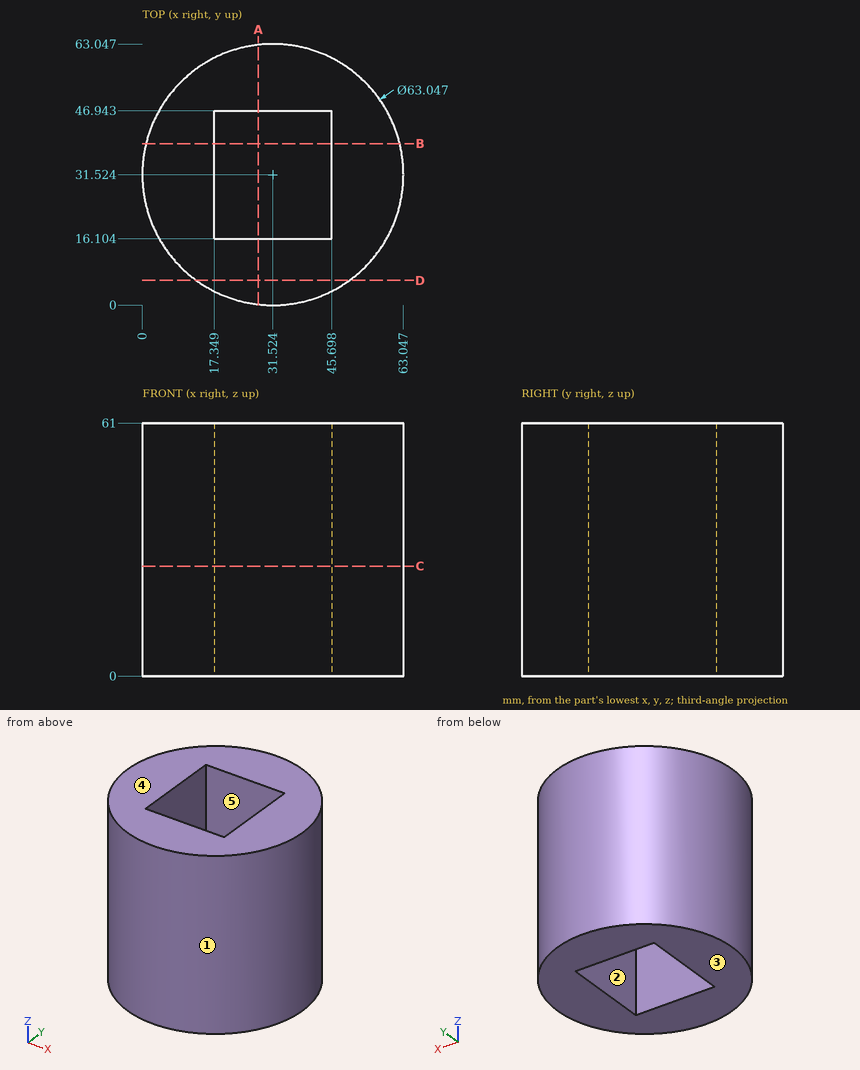
The figure shows three views and two pictorial views of one solid part (mm, origin at its lowest corner). Answer the questions. A direction names the side the tool comes from. Give positions to 0.01 mm unless a question says otherwise; leave off trailing zeros. Write each loop counter-clockwise with the first axis right and the second up, starting at its lowest first coordinate (ties: lowest second). Pieces come first, ordered by that corner, then holes.
Q1. For a pull along Y with two mould halves and no side action, classify the marked faces 1, 2 and 3 as released by +Y, released by -Y, zero draft, split by the parting line, or undercut.
Answer:
face 1: split by the parting line
face 2: undercut
face 3: zero draft
Q2. The part is cut by section B-B on y = 39. Give the vertices of the cut face in (x, z).
Answer:
outline: (0.9, 0) - (17.35, 0) - (17.35, 61) - (0.9, 61) - close; (45.7, 0) - (62.15, 0) - (62.15, 61) - (45.7, 61) - close
Q3. Given pin 1 (6 mm diameter, centred on x = 28, z = 30.5, fed in from -Y); pin 2 (2 mm diameter, centred on x = 53, y = 6.5, fed in from +Z); pin 3 (8.5 mm diameter, centred on x = 28.5, z = 24, fed in from +Y); pin 4 (1 mm diameter, centred on y = 56.5, z = 32, fed in from -X), each flat-ended and moving along its own axis, determine where each tip first touches the part or whether it passes through.
Answer:
pin 1: stops at y = 0
pin 2: passes through
pin 3: stops at y = 63.05
pin 4: stops at x = 11.66
Q4. Straight lines are drawn through the part: L1, parallel to Y at x = 39.5, z = 17.5 (1 decimal); L2, parallel to X at y = 8, z = 46.5; L3, parallel to X at y = 28, z = 3. For each, find the intervals that lie inside material, in ascending order.
Answer:
L1: y = 1 to 16.1, 46.9 to 62
L2: x = 10.54 to 52.51
L3: x = 0.2 to 17.35, 45.7 to 62.85
Q5. The part is cut by section C-C on z = 26.5. Give the vertices of the cut face in (x, y).
Answer:
outline: circle Ø63.05 at (31.52, 31.52); hole (17.35, 16.1) - (45.7, 16.1) - (45.7, 46.94) - (17.35, 46.94) - close
Q6. A tool of negligible diameter and unlimited length cuts with its end or side. For the marked faces 4 and 5, from which of +Z, -Z, +X, -X, +Y, -Y can it reach the whole face along a straight path? Write none if from no direction.
Answer:
face 4: +Z, +X, -X, +Y, -Y
face 5: +Z, -Z
Q7. The part is cut by section A-A on x = 28. Give the vertices of the cut face in (y, z), and give its area (3 significant figures).
Answer:
outline: (0.2, 0) - (16.1, 0) - (16.1, 61) - (0.2, 61) - close; (46.94, 0) - (62.85, 0) - (62.85, 61) - (46.94, 61) - close
area: 1,940 mm2
Q8. The part is cut by section D-D on y = 6. Give the vertices of the cut face in (x, z) (1 decimal).
Answer:
outline: (13, 0) - (50, 0) - (50, 61) - (13, 61) - close
